Autodesk Inventor part; units mm, degrees
ref_plane "YZ Plane" through (0, 0, 0) normal (1, 0, 0) x (0, 1, 0)
ref_plane "XZ Plane" through (0, 0, 0) normal (0, 1, 0) x (-1, 0, 0)
ref_plane "XY Plane" through (0, 0, 0) normal (0, 0, 1) x (1, 0, 0)
ref_plane "Arbeitsebene1" through (0, 0, 0) normal (0, 0, 1) x (1, 0, 0)
sketch "Skizze1" plane through (0, 0, 0) normal (0, 0, 1) x (1, 0, 0)
  circle A0 centre (-20, -44.9) radius 1.75
  circle A1 centre (30, -44.9) radius 1.75
  circle A2 centre (20, -44.9) radius 1.75
  circle A3 centre (-30, -44.9) radius 1.75
  line L0 (-35, -49.8) -> (-35, -35.9)
  line L1 (35, -49.8) -> (-35, -49.8)
  line L2 (35, -35.9) -> (35, -49.8)
  line L3 (-35, -35.9) -> (35, -35.9)
  arc A4 (-19.0986, 43.4) -> (-20.9014, 43.4) centre (-20, 44.9) ccw
  line L4 (19.0986, 43.4) -> (-19.0986, 43.4)
  arc A5 (20.9014, 43.4) -> (19.0986, 43.4) centre (20, 44.9) ccw
  line L5 (29.0986, 43.4) -> (20.9014, 43.4)
  arc A6 (30.9014, 43.4) -> (29.0986, 43.4) centre (30, 44.9) ccw
  line L6 (35, 43.4) -> (30.9014, 43.4)
  line L7 (35, 49.8) -> (35, 43.4)
  line L8 (-35, 49.8) -> (35, 49.8)
  line L9 (-35, 43.4) -> (-35, 49.8)
  line L10 (-30.9014, 43.4) -> (-35, 43.4)
  arc A7 (-29.0986, 43.4) -> (-30.9014, 43.4) centre (-30, 44.9) ccw
  line L11 (-20.9014, 43.4) -> (-29.0986, 43.4)
  line L12 (35, -49.8) -> (-35, -49.8)
  line L13 (-35, -49.8) -> (-35, 49.8)
  line L14 (-35, 49.8) -> (35, 49.8)
  line L15 (35, 49.8) -> (35, -49.8)
  point P0 (0, 0)
extrude "Extrusion1" add sketch "Skizze1" along normal blind 3 contours A0 | A1 | A2 | A3 | L0 L3 L2 L1 | L13 L10 A7 L11 A4 L4 A5 L5 A6 L6 L15 L3 | L9 L8 L7 L6 A6 L5 A5 L4 A4 L11 A7 L10
sketch "Skizze2" plane through (0, 0, 3) normal (0, 0, 1) x (1, 0, 0)
  circle A0 centre (30, -44.9) radius 1.75
  circle A1 centre (20, -44.9) radius 1.75
  circle A2 centre (-20, -44.9) radius 1.75
  circle A3 centre (-30, -44.9) radius 1.75
  arc A4 (30.9014, 43.4) -> (29.0986, 43.4) centre (30, 44.9) ccw
  arc A5 (20.9014, 43.4) -> (19.0986, 43.4) centre (20, 44.9) ccw
  arc A6 (-19.0986, 43.4) -> (-20.9014, 43.4) centre (-20, 44.9) ccw
  arc A7 (-29.0986, 43.4) -> (-30.9014, 43.4) centre (-30, 44.9) ccw
  point P0 (0, 0)
hole "Bohrung1" at (30, 44.9, 3) at (20, 44.9, 3) at (-30, -44.9, 3) at (-20, -44.9, 3) at (20, -44.9, 3) at (30, -44.9, 3) at (-20, 44.9, 3) at (-30, 44.9, 3) direction (0, 0, -1) diameter 2.9 end through all
properties part number "20_Projector_Sony_Moun_2"
The model under review builds one solid part; all positions refer to its coordinate system, in mm. Round coordinates to 2 decimals unless told otherwise and drop trailing zeros. Order: outer loops, then holes, each group sorted by start corner. A loop starts at its lowest first (then second) coordinate and runs counter-clockwise, first axis right, second up. Notation, with made-up numbers: (69.5, 30.5) - (80.5, 30.5) arc R17 ccw to (80.5, 40.5) - close; hole circle Ø6 at (-15, -25). An arc over 180 degrees is marked (long way). Use one line per item in the form item = value.
Q1. Add section A-A on x = 20. Give the boundary of the cut face in (y, z).
Response values:
outline = (-49.8, 0) - (-46.35, 0) - (-46.35, 3) - (-49.8, 3) - close; (-43.45, 0) - (43.45, 0) - (43.45, 3) - (-43.45, 3) - close; (46.35, 0) - (49.8, 0) - (49.8, 3) - (46.35, 3) - close
Q2. Add section B-B on y = 44.9. Give the boundary of the cut face in (x, z).
Response values:
outline = (-35, 0) - (-31.45, 0) - (-31.45, 3) - (-35, 3) - close; (-28.55, 0) - (-21.45, 0) - (-21.45, 3) - (-28.55, 3) - close; (-18.55, 0) - (18.55, 0) - (18.55, 3) - (-18.55, 3) - close; (21.45, 0) - (28.55, 0) - (28.55, 3) - (21.45, 3) - close; (31.45, 0) - (35, 0) - (35, 3) - (31.45, 3) - close
Q3. To check wall thickness, follow line 1 (Y direction, x = -20, z = 2.8); line 2 (X direction, y = 44.9, z = 1.1). State the ranges of each line that lie inside material, in increasing order.
Response values:
line_1 = -49.8 to -46.35, -43.45 to 43.45, 46.35 to 49.8
line_2 = -35 to -31.45, -28.55 to -21.45, -18.55 to 18.55, 21.45 to 28.55, 31.45 to 35
Q4. Mouldability with a two-part tool opening along Y and no side actions: class faces 1 (the cylindrical face through (-20.06, 46.35, 1.48)), 2 (the flat face through (0, 49.8, 1)), 3 (the flat face through (-35, -1, 1)), 4 (the cylindrical face through (30.88, 46.05, 1.48)) as pulls with the +Y half, pulls with the -Y half, needs draft (parallel to the pull), parting line crosses it, or undercut.
Response values:
face_1 = undercut
face_2 = pulls with the +Y half
face_3 = needs draft
face_4 = undercut
